Can you work these out from the drawing? Everything is in mm from the part's minimum corner. Coordinates: 2 decimals unless noted, no trailing zeros. Loops run counter-clockwise (first coordinate to the right, second up) from the corner with the lowest first, then second, coordinate; pieces in that order, holes last. Notation, with made-up numbers: M -12,47.5 L 38,47.5 A19 cw 38,81.5 Z; hole C -39,22.5 d4. An arc over 180 degrees is marked long. Write each question's results on one line, items separated by ' | '.
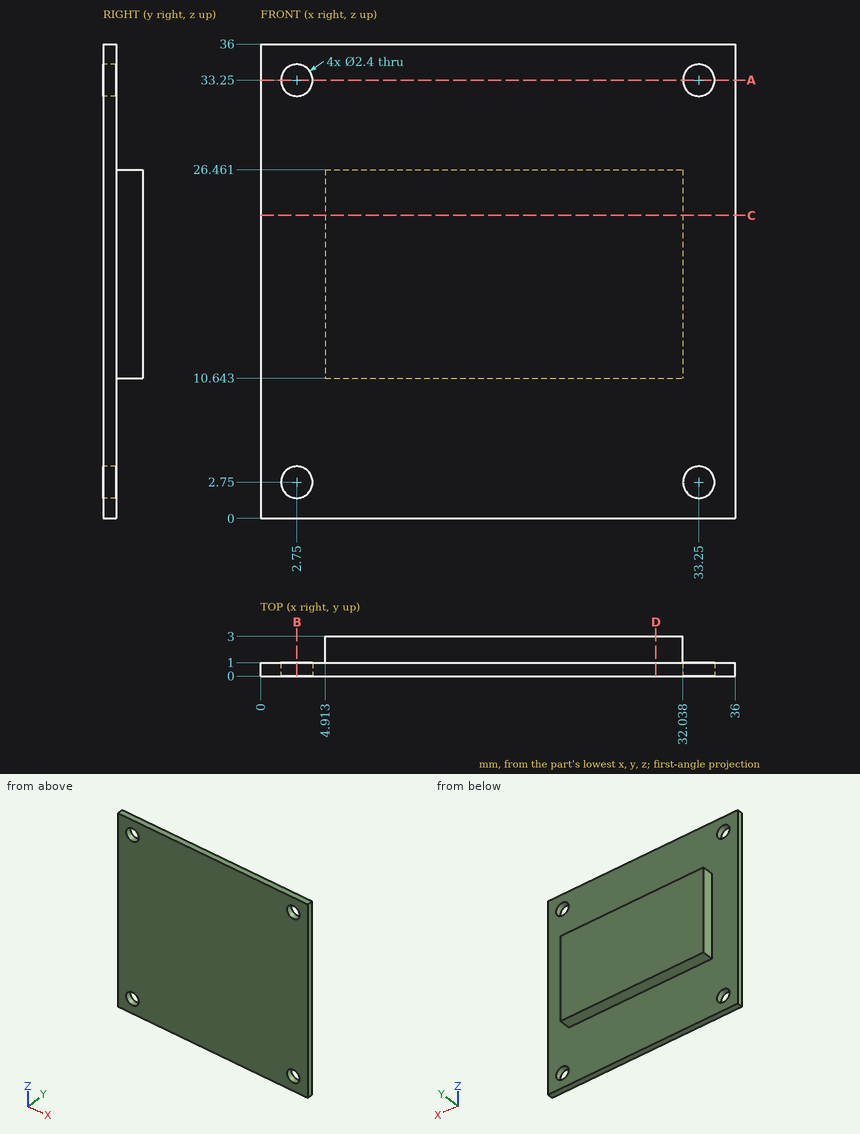
(1) Will these pins go through, and if not, where does the flat tip stop? P1, Ø3, axis at x = 33.25, z = 33.25, coming from the -Y side; P2, Ø1, axis at x = 17, y = 2, coming from the -Z side; P3, Ø2, axis at x = 2.75, z = 33.25, coming from the -Y side; P4, Ø1, axis at y = 2, z = 14.5, coming from the -X side.
Reported:
P1: stops at y = 0 | P2: stops at z = 10.64 | P3: passes through | P4: stops at x = 4.91
(2) Imagine slicing it at A-A, the plane z = 33.25. List the corners of the cut face in (x, y) for me.
Reported:
outline: M 0,0 L 1.55,0 L 1.55,1 L 0,1 Z; M 3.95,0 L 32.05,0 L 32.05,1 L 3.95,1 Z; M 34.45,0 L 36,0 L 36,1 L 34.45,1 Z
(3) Please list where these lines run through material, in increasing order: probe 1 along Z at (x, y) = (33.25, 0.3); probe 2 along Z at (x, y) = (31, 2.9). Write a range as from..to.
Reported:
probe 1: z = 0..1.55, 3.95..32.05, 34.45..36 | probe 2: z = 10.64..26.46
(4) Imagine slicing it at B-B, the plane x = 2.75. List the corners of the cut face in (y, z) for me.
Reported:
outline: M 0,0 L 1,0 L 1,1.55 L 0,1.55 Z; M 0,3.95 L 1,3.95 L 1,32.05 L 0,32.05 Z; M 0,34.45 L 1,34.45 L 1,36 L 0,36 Z
(5) Imagine slicing it at C-C, the plane z = 23. List the corners of the cut face in (x, y) for me.
Reported:
outline: M 0,0 L 36,0 L 36,1 L 32.04,1 L 32.04,3 L 4.91,3 L 4.91,1 L 0,1 Z
(6) Imagine slicing it at D-D, the plane x = 30. List the corners of the cut face in (y, z) for me.
Reported:
outline: M 0,0 L 1,0 L 1,10.64 L 3,10.64 L 3,26.46 L 1,26.46 L 1,36 L 0,36 Z
